Model file for the job. Use its own axes, mm. Face numbers are marked on the shaded views. A direction names the side the tool comes from. Round coordinates to 2 decimals unless told otherwise and drop trailing zeros. Loops run counter-clockwise (first coordinate to the right, second up) from the corner with the lowest first, then second, coordinate; pieces in that order, holes last. Notation, with made-up numbers: (74, 47) -> (105, 47) arc R24 cw to (105, 81) -> close; hole circle Ø1 at (-32, 29). An arc over 180 degrees is marked (long way). Use a Markdown table: item, result. Add a question column.
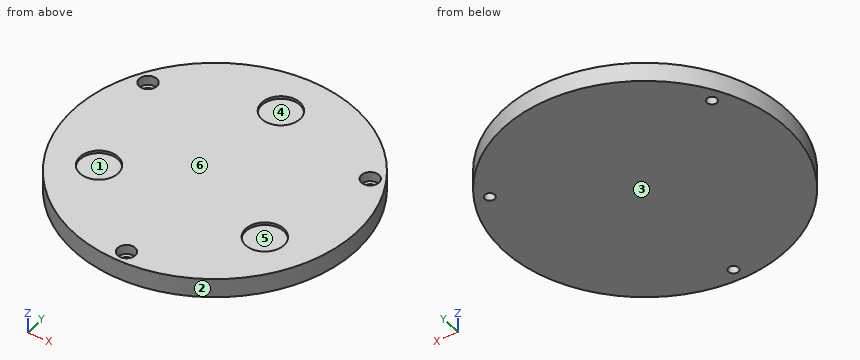
```python
from build123d import *

# Parameters (mm, degrees)
F0_R     = 46.99
F1_DEPTH = 6.35
F2_R     = 6.35
F3_DEPTH = 0.9144
F4_R     = 2.921
F5_DEPTH = 3.175
F6_R     = 1.65
F7_DEPTH = 25.4


with BuildPart() as f1:
    # F0 (on Top) → F1 (new body)
    with BuildSketch(Plane.XY):
        Circle(F0_R)
    extrude(amount=F1_DEPTH)

    # F2 (on face) → F3 (cut)
    with BuildSketch(Plane.XY.offset(6.35)):
        with Locations((0, 31.75)):
            Circle(F2_R)
        with Locations((-27.496307, -15.875)):
            Circle(F2_R)
        with Locations((27.496307, -15.875)):
            Circle(F2_R)
    extrude(amount=-F3_DEPTH, mode=Mode.SUBTRACT)

    # F4 (on face) → F5 (cut)
    with BuildSketch(Plane.XY.offset(6.35)):
        with Locations((0, -42.545)):
            Circle(F4_R)
        with Locations((-36.845051, 21.2725)):
            Circle(F4_R)
        with Locations((36.845051, 21.2725)):
            Circle(F4_R)
    extrude(amount=-F5_DEPTH, mode=Mode.SUBTRACT)

    # F6 (on face) → F7 (cut)
    with BuildSketch(Plane.XY.offset(6.35)):
        with Locations((-36.845051, 21.2725)):
            Circle(F6_R)
        with Locations((36.845051, 21.2725)):
            Circle(F6_R)
        with Locations((0, -42.545)):
            Circle(F6_R)
    extrude(amount=-F7_DEPTH, mode=Mode.SUBTRACT)


solid = f1.part
```
1) Wall check: probe 1 along Y at (x, z) = (0, 4.6); probe 2 along Y at (x, z) = (-35, 4.75); probe 3 along X at (y, z) = (-25, 5.5). Give the ranges that are in metal, low to high. Write a range as from..to.
2) Pull direction Y, two halves, no side cores. Call the marked faces 1, 2, 3 and 4: +Y half, -Y half, draft (parallel to the pull), parting line (faces both ways), or undercut.
3) Cut at C-C on x = 29.5. Write the cut outline in (y, z).
4) Pin check, flat tips, straight feed: pin 1 Ø2 at (x, y) = (36.85, 21.27) entering from +Z; pin 2 Ø1.5 at (y, z) = (-29.5, 1.5) entering from +X; pin 3 Ø4 at (x, y) = (1, 35) entering from +Z; pin 4 Ø5.5 at (x, y) = (0, -42.545) entering from +Z (3 decimals). Stop position of each tip, or through.
5) Cut at A-A on x = 0. Write the cut outline in (y, z) (3 decimals), and give its area (3 significant figures).
6) Cut at D-D on z = 2. Count the separate pieces of the cut face and the enclosed holes in it, and give its area (3 significant figures).
7) Cut at B-B on y = 37. Write the cut outline in (x, z), and give its area (3 significant figures).
8) Tool access for the marked faces 5 and 6: list every direction of +Z, -Z, +X, -X, +Y, -Y with a clear straight run to the whole face (end or side of a thin tool).
Established:
| question | item | result |
|---|---|---|
| 1 | probe 1 | y = -46.99..-45.47, -39.62..46.99 |
| 1 | probe 2 | y = -31.35..19.01, 23.54..31.35 |
| 1 | probe 3 | x = -39.79..39.79 |
| 2 | face 1 | undercut |
| 2 | face 2 | parting line |
| 2 | face 3 | draft |
| 2 | face 4 | undercut |
| 3 | outline | (-36.58, 0) -> (36.58, 0) -> (36.58, 6.35) -> (-9.85, 6.35) -> (-9.85, 5.44) -> (-21.9, 5.44) -> (-21.9, 6.35) -> (-36.58, 6.35) -> close |
| 4 | pin 1 | passes through |
| 4 | pin 2 | stops at x = 37.17 |
| 4 | pin 3 | stops at z = 5.44 |
| 4 | pin 4 | stops at z = 3.175 |
| 5 | outline | (-46.99, 0) -> (-44.195, 0) -> (-44.195, 3.175) -> (-45.466, 3.175) -> (-45.466, 6.35) -> (-46.99, 6.35) -> close; (-40.895, 0) -> (46.99, 0) -> (46.99, 6.35) -> (38.1, 6.35) -> (38.1, 5.436) -> (25.4, 5.436) -> (25.4, 6.35) -> (-39.624, 6.35) -> (-39.624, 3.175) -> (-40.895, 3.175) -> close |
| 5 | area | 556 mm^2 |
| 6 | separate pieces | 1 |
| 6 | enclosed holes | 3 |
| 6 | area | 6,910 mm^2 |
| 7 | outline | (-28.97, 0) -> (28.97, 0) -> (28.97, 6.35) -> (3.57, 6.35) -> (3.57, 5.44) -> (-3.57, 5.44) -> (-3.57, 6.35) -> (-28.97, 6.35) -> close |
| 7 | area | 361 mm^2 |
| 8 | face 5 | +Z |
| 8 | face 6 | +Z, +X, -X, +Y, -Y |
